```python
from build123d import *

# Parameters (mm, degrees)
SKETCH1_W           = 101.6
SKETCH1_H           = 101.6
BOSS_EXTRUDE1_DEPTH = 12.7
SKETCH3_R           = 2.2479
SKETCH3_R_2         = 1.7272
CUT_EXTRUDE1_DEPTH  = 73.955945611


with BuildPart() as part:
    # Sketch1 → Boss-Extrude1 (new body)
    with BuildSketch(Plane(origin=(0, 0, 0), x_dir=(1, 0, 0), z_dir=(0, 1, 0))):
        Rectangle(SKETCH1_W, SKETCH1_H)
    extrude(amount=-BOSS_EXTRUDE1_DEPTH)

    # Sketch3 → Cut-Extrude1 (cut, through all)
    with BuildSketch(Plane(origin=(0, 0, 0), x_dir=(1, 0, 0), z_dir=(0, 1, 0))):
        with Locations(Location((-41.819743879, 41.819743879, 0), (0, 0, 270))):
            Circle(SKETCH3_R)
        with Locations(Location((41.819743879, 41.819743879, 0), (0, 0, 270))):
            Circle(SKETCH3_R)
        with Locations(Location((41.819743879, -41.819743879, 0), (0, 0, 270))):
            Circle(SKETCH3_R)
        with Locations(Location((-41.819743879, -41.819743879, 0), (0, 0, 270))):
            Circle(SKETCH3_R)
        with Locations(Location((0, 0, 0), (0, 0, 270))):
            Circle(SKETCH3_R_2)
    extrude(amount=-CUT_EXTRUDE1_DEPTH, mode=Mode.SUBTRACT)


solid = part.part
```
The model under review builds one solid part; all positions refer to its coordinate system, in mm. Round coordinates to 2 decimals unless told otherwise and drop trailing zeros. Loops run counter-clockwise (first coordinate to the right, second up) from the corner with the lowest first, then second, coordinate; pieces in that order, holes last. Notation, with made-up numbers: M 88.5,58.25 L 121.5,58.25 A25 ccw 121.5,95.25 Z; hole C 88,-31 d7. An arc over 180 degrees is marked long. Write item = value, one per line.
Item 1: Take a section at A-A on z = 0. Write out the cut boundary in (x, y), then the cut area to 3 significant figures.
Return value:
outline = M -50.8,-12.7 L -1.73,-12.7 L -1.73,0 L -50.8,0 Z; M 1.73,-12.7 L 50.8,-12.7 L 50.8,0 L 1.73,0 Z
area = 1,250 mm2
Item 2: For line 1 (Z direction, x = 42, y = -11.5); line 2 (X direction, y = -11, z = 41.5), list the stretches that pass through material, from the lowest coordinate up. Write a range as [from, to].
Return value:
line_1 = [-50.8, -44.06], [-39.58, 39.58], [44.06, 50.8]
line_2 = [-50.8, -44.04], [-39.59, 39.59], [44.04, 50.8]
Item 3: The part is to be moulded in two halves that separate along Z. For faces 1 (the cylindrical face through (-43.19, -6.26, -43.6)), 2 (the flat face through (-1, -6, 50.8)), 3 (the flat face through (50.8, -6, 1)), say which applies: released by +Z, released by -Z, zero draft, split by the parting line, or undercut.
Return value:
face_1 = undercut
face_2 = released by +Z
face_3 = zero draft
Item 4: Insertion check: P1, Ø2.5, axis at x = 41.82, z = 41.82, coming from the -Y side. The pin has a flat end and moves straight along its axis. Give the tip position at first contact, or say it passes through.
Return value:
P1 = through
Item 5: Take a section at B-B on x = 0. Write out the cut boundary in (y, z).
Return value:
outline = M -12.7,-50.8 L 0,-50.8 L 0,-1.73 L -12.7,-1.73 Z; M -12.7,1.73 L 0,1.73 L 0,50.8 L -12.7,50.8 Z
